For this review, take the finished solid that the model builds, in its own axes (mm). A direction names the side the tool comes from. Round coordinates to 2 decimals unless told otherwise and drop trailing zeros. Loops run counter-clockwise (first coordinate to the right, second up) from the corner with the lowest first, then second, coordinate; pieces in that order, holes last.
```python
from build123d import *

# Parameters (mm, degrees)
BOSS_EXTRUDE1_DEPTH = 25.4
SKETCH2_R           = 42.50055
CUT_EXTRUDE1_DEPTH  = 44.45
SKETCH3_R           = 39.37
CUT_EXTRUDE2_DEPTH  = 31.75
SKETCH4_R           = 6.35
CUT_EXTRUDE3_DEPTH  = 19.05
CUT_EXTRUDE4_START  = -19.05
SKETCH5_R           = 6.35
CUT_EXTRUDE4_DEPTH  = 19.05
SKETCH6_R           = 6.35
CUT_EXTRUDE5_DEPTH  = 19.05
CUT_EXTRUDE6_START  = -19.05
SKETCH7_R           = 6.35
CUT_EXTRUDE6_DEPTH  = 19.05


with BuildPart() as part:
    # Sketch1 → Boss-Extrude1 (new, symmetric)
    with BuildSketch(Plane.XY):
        with BuildLine():
            Line((-107.95, -76.2), (107.95, -76.2))
            ThreePointArc((107.95, -76.2), (112.440128061, -74.340128061), (114.3, -69.85))
            Line((114.3, -69.85), (114.3, 69.85))
            ThreePointArc((114.3, 69.85), (112.440128061, 74.340128061), (107.95, 76.2))
            Line((107.95, 76.2), (-107.95, 76.2))
            ThreePointArc((-107.95, 76.2), (-112.440128061, 74.340128061), (-114.3, 69.85))
            Line((-114.3, 69.85), (-114.3, -69.85))
            ThreePointArc((-114.3, -69.85), (-112.440128061, -74.340128061), (-107.95, -76.2))
        make_face()
    extrude(amount=BOSS_EXTRUDE1_DEPTH, both=True)

    # Sketch2 → Cut-Extrude1 (cut)
    with BuildSketch(Plane.XY.offset(25.4)):
        Circle(SKETCH2_R)
    extrude(amount=-CUT_EXTRUDE1_DEPTH, mode=Mode.SUBTRACT)

    # Sketch3 → Cut-Extrude2 (cut)
    with BuildSketch(Plane.XY.offset(-19.05)):
        Circle(SKETCH3_R)
    extrude(amount=-CUT_EXTRUDE2_DEPTH, mode=Mode.SUBTRACT)

    # Sketch4 → Cut-Extrude3 (cut)
    with BuildSketch(Plane(origin=(0, 76.2, 0), x_dir=(1, 0, 0), z_dir=(0, 1, 0))):
        with Locations(Location((-63.5, 0, 0), (0, 0, 270))):
            Circle(SKETCH4_R)
        with Locations(Location((63.5, 0, 0), (0, 0, 270))):
            Circle(SKETCH4_R)
    extrude(amount=-CUT_EXTRUDE3_DEPTH, mode=Mode.SUBTRACT)

    # Sketch5 → Cut-Extrude4 (cut)
    with BuildSketch(Plane.XZ.offset(76.2).offset(CUT_EXTRUDE4_START)):
        with Locations(Location((-63.5, 0, 0), (0, 0, 90))):
            Circle(SKETCH5_R)
        with Locations(Location((63.5, 0, 0), (0, 0, 90))):
            Circle(SKETCH5_R)
    extrude(amount=CUT_EXTRUDE4_DEPTH, mode=Mode.SUBTRACT)

    # Sketch6 → Cut-Extrude5 (cut)
    with BuildSketch(Plane(origin=(114.3, 0, 0), x_dir=(0, 0, -1), z_dir=(1, 0, 0))):
        with Locations((0, 50.8)):
            Circle(SKETCH6_R)
        with Locations((0, -50.8)):
            Circle(SKETCH6_R)
    extrude(amount=-CUT_EXTRUDE5_DEPTH, mode=Mode.SUBTRACT)

    # Sketch7 → Cut-Extrude6 (cut)
    with BuildSketch(Plane.ZY.offset(114.3).offset(CUT_EXTRUDE6_START)):
        with Locations(Location((0, 50.8, 0), (0, 0, 180))):
            Circle(SKETCH7_R)
        with Locations(Location((0, -50.8, 0), (0, 0, 180))):
            Circle(SKETCH7_R)
    extrude(amount=CUT_EXTRUDE6_DEPTH, mode=Mode.SUBTRACT)


solid = part.part
```
(1) The part is to be moulded in two halves that separate along Y. For faces 1 (the flat face through (64, 57.15, 0)), 2 (the flat face through (-95.25, -51, 0)), 3 (the cylindrical face through (69.7, -66.54, -1.38)), say which applies: pulls with the +Y half, pulls with the -Y half, needs draft (parallel to the pull), parting line crosses it, or undercut.
(2) For L1, parallel to X at y = 62, z = 0.5; L2, parallel to Z at x = -104, y = 50; L3, parallel to Y at x = 0, z = 9, list the stretches that pass through material, from the lowest coordinate up.
(3) Add section D-D (x = 0). Give the boundary of the cut face in (y, z).
(4) Add section B-B (z = 13.5). Give the boundary of the cut face in (x, y).
(5) For faces 4 (the flat face through (95.25, -51, 0)), 5 (the flat face through (-64, -57.15, 0)), 6 (the cylindrical face through (-69.7, 66.81, -1.38)), 7 (the cylindrical face through (-104.6, -57.1, 0.8)), list the 3-axis set-ups (+Z, -Z, +X, -X, +Y, -Y) from which the entire face can be reached by the end or side of a thin tool; tool diameter is ignored.
(6) Insertion check: pin 1 Ø7.5 at (x, z) = (63.5, 0) entering from +Y; pin 2 Ø7.5 at (y, z) = (50.8, 0) entering from -X; pin 3 Ø6.5 at (y, z) = (48, -0.5) entering from +X. Each pin has a flat end and moves straight along its axis. Give the tip position at first contact, or say it passes through.
(7) Add section C-C (x = -63.5). Give the boundary of the cut face in (y, z), plus the area to 3 significant figures.
(8) Add section A-A (y = 0). Give the boundary of the cut face in (x, z).
Outcome:
1. face 1: pulls with the +Y half
1. face 2: undercut
1. face 3: needs draft
2. L1: x = -114.3 to -69.83, -57.17 to 57.17, 69.83 to 114.3
2. L2: z = -25.4 to -6.3, 6.3 to 25.4
2. L3: y = -76.2 to -42.5, 42.5 to 76.2
3. outline: (-76.2, -25.4) - (-39.37, -25.4) - (-39.37, -19.05) - (-42.5, -19.05) - (-42.5, 25.4) - (-76.2, 25.4) - close; (39.37, -25.4) - (76.2, -25.4) - (76.2, 25.4) - (42.5, 25.4) - (42.5, -19.05) - (39.37, -19.05) - close
4. outline: (-114.3, -69.85) arc R6.35 ccw to (-107.95, -76.2) - (107.95, -76.2) arc R6.35 ccw to (114.3, -69.85) - (114.3, 69.85) arc R6.35 ccw to (107.95, 76.2) - (-107.95, 76.2) arc R6.35 ccw to (-114.3, 69.85) - close; hole circle Ø85 at (0, 0)
5. face 4: +X
5. face 5: -Y
5. face 6: +Y
5. face 7: -X
6. pin 1: stops at y = 57.15
6. pin 2: stops at x = -95.25
6. pin 3: stops at x = 95.25
7. outline: (-76.2, -25.4) - (76.2, -25.4) - (76.2, -6.35) - (57.15, -6.35) - (57.15, 6.35) - (76.2, 6.35) - (76.2, 25.4) - (-76.2, 25.4) - (-76.2, 6.35) - (-57.15, 6.35) - (-57.15, -6.35) - (-76.2, -6.35) - close
7. area: 7,260 mm2
8. outline: (-114.3, -25.4) - (-39.37, -25.4) - (-39.37, -19.05) - (-42.5, -19.05) - (-42.5, 25.4) - (-114.3, 25.4) - close; (39.37, -25.4) - (114.3, -25.4) - (114.3, 25.4) - (42.5, 25.4) - (42.5, -19.05) - (39.37, -19.05) - close
